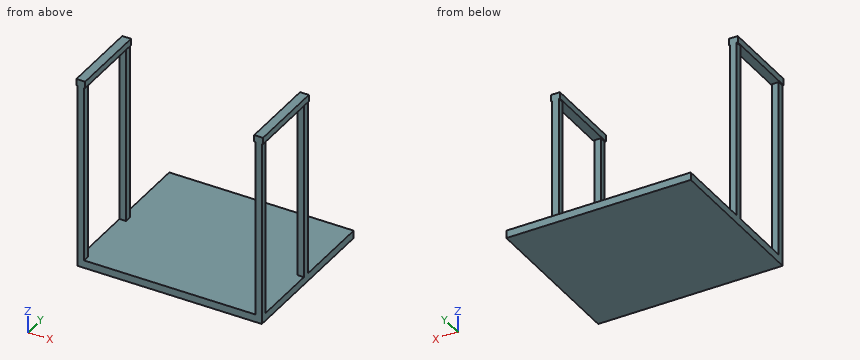
```python
from build123d import *

# Parameters (mm, degrees)
F0_W     = 533.4
F0_H     = 457.2
F1_DEPTH = 44.45
F2_W     = 38.1
F2_H     = 38.1
F3_DEPTH = 1066.8
F4_W     = 50.8
F4_H     = 457.2
F5_DEPTH = 38.1
F6_ANGLE = 180


with BuildPart() as f1:
    # F0 (on Top) → F1 (new body)
    with BuildSketch(Plane.XY):
        with Locations((-266.7, 228.6)):
            Rectangle(F0_W, F0_H)
        with Locations((266.7, 228.6)):
            Rectangle(F0_W, F0_H)
        with Locations((-266.7, -228.6)):
            Rectangle(F0_W, F0_H)
        with Locations((266.7, -228.6)):
            Rectangle(F0_W, F0_H)
    extrude(amount=F1_DEPTH)

    # F2 (on face) → F3 (join)
    with BuildSketch(Plane.XY.offset(44.45)):
        with Locations((-514.35, 438.15)):
            Rectangle(F2_W, F2_H)
        with Locations((514.35, 438.15)):
            Rectangle(F2_W, F2_H)
        with Locations((-514.35, 19.05)):
            Rectangle(F2_W, F2_H)
        with Locations((514.35, 19.05)):
            Rectangle(F2_W, F2_H)
    extrude(amount=F3_DEPTH)

    # F4 (on face) → F5 (join)
    with BuildSketch(Plane.XY.offset(1111.25)):
        with Locations((-514.35, 228.6)):
            Rectangle(F4_W, F4_H)
        with Locations((514.35, 228.6)):
            Rectangle(F4_W, F4_H)
    extrude(amount=-F5_DEPTH)


with BuildPart() as f1_1:
    # F6: moved
    add(f1.part.rotate(Axis((-533.4, -457.2, 22.225), (0, 0, 1)), F6_ANGLE))


with BuildPart() as f1_2:
    # F7: moved
    add(f1_1.part.moved(Location((1155.7, 833.12, 0))))


solid = f1_2.part
```
Check sheet for the modelled part. Datum: model origin and axes. Units: mm. Coordinates: 2 decimals unless noted, no trailing zeros. Order: outer loops, then holes, each group sorted by start corner. A loop starts at its lowest first (then second) coordinate and runs counter-clockwise, first axis right, second up. Notation, with made-up numbers: M 51,32.25 L 66,32.25 A21 ccw 66,50.25 Z; hole C 84,2 d7. An arc over 180 degrees is marked long. One line per question, with ' | ' between items. Start each with the question number.
Item 1: Sectioned sample at C-C on x = 499. Record the cut outline in (y, z).
Item 2: Sectioned sample at D-D on y = 68.5. Record the cut outline in (x, z), and give its area (3 significant figures).
Item 3: Sectioned sample at B-B on z = 963. Record the cut outline in (x, y), and give its area (3 significant figures).
Item 4: Sectioned sample at A-A on y = -460. Record the cut outline in (x, z), and give its area (3 significant figures).
Item 5: Material ranges on line 1 (Z direction, x = -220, y = -167), recorded low to high.
Item 6: Gauge pin test, flat ends, axial feed: P1, Ø19, axis at x = 595, z = 755.5, coming from the +Y side; P2, Ø11.5, axis at y = -522, z = 439.5, coming from the +X side; P3, Ø11.5, axis at y = -103.5, z = 771, coming from the -X side. Record the tip position at first contact, or that the pin passes through.
Answer below:
1) outline: M -538.48,0 L 375.92,0 L 375.92,44.45 L -538.48,44.45 Z
2) outline: M -444.5,0 L 622.3,0 L 622.3,44.45 L -444.5,44.45 Z | area: 47,400 mm^2
3) outline: M -444.5,-538.48 L -406.4,-538.48 L -406.4,-500.38 L -444.5,-500.38 Z; M -444.5,-119.38 L -406.4,-119.38 L -406.4,-81.28 L -444.5,-81.28 Z; M 584.2,-538.48 L 622.3,-538.48 L 622.3,-500.38 L 584.2,-500.38 Z; M 584.2,-119.38 L 622.3,-119.38 L 622.3,-81.28 L 584.2,-81.28 Z | area: 5,810 mm^2
4) outline: M -450.85,1073.15 L -400.05,1073.15 L -400.05,1111.25 L -450.85,1111.25 Z; M -444.5,0 L 622.3,0 L 622.3,44.45 L -444.5,44.45 Z; M 577.85,1073.15 L 628.65,1073.15 L 628.65,1111.25 L 577.85,1111.25 Z | area: 51,300 mm^2
5) line 1: z = 0 to 44.45
6) P1: stops at y = -81.28 | P2: stops at x = 622.3 | P3: stops at x = -444.5
